Autodesk Inventor part; units mm, degrees
ref_plane "YZ Plane" through (0, 0, 0) normal (1, 0, 0) x (0, 1, 0)
ref_plane "XZ Plane" through (0, 0, 0) normal (0, 1, 0) x (-1, 0, 0)
ref_plane "XY Plane" through (0, 0, 0) normal (0, 0, 1) x (1, 0, 0)
sketch "Sketch1" plane through (0, 0, 0) normal (0, 1, 0) x (-1, 0, 0)
  line L0 (0, 0) -> (49, 0) construction
  line L1 (49, 0) -> (49, -58) construction
  line L2 (49, -58) -> (0, -58) construction
  line L3 (0, -58) -> (0, 0) construction
  line L4 (53.5, 32) -> (-4.5, 32) construction
  line L5 (-4.5, 32) -> (-4.5, -62) construction
  line L6 (-4.5, -62) -> (53.5, -62) construction
  line L7 (53.5, -62) -> (53.5, 32) construction
  line L8 (53.5, -58) -> (-4.5, -58) construction
  line L9 (24.5, -62) -> (24.5, -133) construction
  line L10 (49, -70.5) -> (28, -70.5) construction
  line L11 (28, -70.5) -> (28, -127.5) construction
  line L12 (28, -127.5) -> (49, -127.5) construction
  line L13 (49, -127.5) -> (49, -70.5) construction
  line L14 (24.5, -99) -> (28, -99) construction
  line L15 (45.5, -127.5) -> (31.5, -127.5) construction
  line L16 (31.5, -127.5) -> (31.5, -140.5) construction
  line L17 (31.5, -140.5) -> (45.5, -140.5) construction
  line L18 (45.5, -140.5) -> (45.5, -127.5) construction
  line L19 (16.5, -82.13) -> (0, -82.13) construction
  line L20 (0, -82.13) -> (0, -112.87) construction
  line L21 (0, -112.87) -> (16.5, -112.87) construction
  line L22 (16.5, -112.87) -> (16.5, -82.13) construction
  line L23 (24.5, -97.5) -> (16.5, -97.5) construction
  circle A0 centre (49, -127.5) radius 1.5
  circle A1 centre (49, -70.5) radius 1.5
  circle A2 centre (28, -70.5) radius 1.5
  circle A3 centre (28, -127.5) radius 1.5
  circle A4 centre (49, -58) radius 1.5
  circle A5 centre (0, -58) radius 1.5
  circle A6 centre (0, 0) radius 1.5
  circle A7 centre (49, 0) radius 1.5
  circle A8 centre (16.5, -82.13) radius 1.5
  circle A9 centre (0, -112.87) radius 1.5
  line L24 (53.5, 32) -> (-4.5, 32) construction
  line L25 (-4.5, 32) -> (-4.5, -140.5) construction
  line L26 (-4.5, -140.5) -> (53.5, -140.5) construction
  line L27 (53.5, -140.5) -> (53.5, 32) construction
  line L28 (56.5, 35) -> (-7.5, 35) construction
  line L29 (-7.5, 35) -> (-7.5, -143.5)
  line L30 (-7.5, -143.5) -> (56.5, -143.5) construction
  line L31 (56.5, -143.5) -> (56.5, 35)
  arc A10 (56.5, 35) -> (-7.5, 35) centre (24.5, 35) ccw
  arc A11 (-7.5, -143.5) -> (56.5, -143.5) centre (24.5, -143.5) ccw
  point P0 (24.5, -58)
  point P1 (38.5, -127.5)
  point P2 (38.5, -140.5)
  point P3 (53.5, -15)
  point P4 (-4.5, -15)
  point P5 (24.5, 32)
  dimension "d0" = 49
  dimension "d1" = 58
  dimension "d2" = 58
  dimension "d3" = 94
  dimension "d7" = 71
  dimension "d8" = 21
  dimension "d9" = 57
  dimension "d10" = 37
  dimension "d11" = 3.5
  dimension "d12" = 14
  dimension "d13" = 13
  dimension "d14" = 16.5
  dimension "d15" = 30.74
  dimension "d16" = 8
  dimension "d17" = 3
  dimension "d18" = 3
  dimension "d19" = 3
  dimension "d20" = 3
  dimension "d21" = 3
  dimension "d22" = 3
  dimension "d23" = 3
  dimension "d24" = 3
  dimension "d25" = 3
  dimension "d26" = 3
  dimension "d27" = 3
  dimension "d43" = 4
extrude "Extrusion1" add sketch "Sketch1" along normal blind 3
sketch "Sketch2" plane through (0, 0, 0) normal (0, -1, 0) x (1, 0, 0)
  arc A0 (-56.5, -143.5) -> (7.5, -143.5) centre (-24.5, -143.5) ccw
  line L0 (7.5, 35) -> (7.5, -143.5)
  arc A1 (7.5, 35) -> (-56.5, 35) centre (-24.5, 35) ccw
  line L1 (-56.5, -143.5) -> (-56.5, 35)
  circle A2 centre (0, -112.87) radius 1.5
  circle A3 centre (-49, 0) radius 1.5
  circle A4 centre (0, 0) radius 1.5
  circle A5 centre (0, -58) radius 1.5
  circle A6 centre (-49, -58) radius 1.5
  circle A7 centre (-28, -127.5) radius 1.5
  circle A8 centre (-28, -70.5) radius 1.5
  circle A9 centre (-49, -70.5) radius 1.5
  circle A10 centre (-49, -127.5) radius 1.5
  circle A11 centre (-16.5, -82.13) radius 1.5
  circle A12 centre (0, 0) radius 3.5
  circle A13 centre (-49, 0) radius 3.5
  circle A14 centre (-49, -58) radius 3.5
  circle A15 centre (0, -58) radius 3.5
  circle A16 centre (-28, -70.5) radius 3.5
  circle A17 centre (-49, -70.5) radius 3.5
  circle A18 centre (-16.5, -82.13) radius 3.5
  circle A19 centre (0, -112.87) radius 3.5
  circle A20 centre (-28, -127.5) radius 3.5
  circle A21 centre (-49, -127.5) radius 3.5
  dimension "d31" = 2
  dimension "d32" = 2
  dimension "d33" = 2
  dimension "d34" = 2
  dimension "d35" = 2
  dimension "d36" = 2
  dimension "d37" = 2
  dimension "d38" = 2
  dimension "d39" = 2
  dimension "d40" = 2
extrude "Extrusion2" cut sketch "Sketch2" against normal blind 2 contours A12 | A13 | A14 | A15 | A16 | A17 | A18 | A19 | A20 | A21
sketch "Sketch3" plane through (0, 3, 0) normal (0, 1, 0) x (1, 0, 0)
  arc A0 (-56.5, -35) -> (7.5, -35) centre (-24.5, -35) ccw
  circle A1 centre (-24.5, -67) radius 4.9
  arc A2 (7.5, 143.5) -> (-56.5, 143.5) centre (-24.5, 143.5) ccw
  circle A3 centre (-24.5, 175.5) radius 4.9
  point P0 (0, 0)
  point P1 (-29.3856, 175.1248)
  point P2 (-19.6144, 175.1248)
  point P3 (-19.6144, -66.6248)
  point P4 (-29.3856, -66.6248)
  dimension "d44" = 9.8
  dimension "d45" = 9.8
extrude "Extrusion3" cut sketch "Sketch3" against normal through all contours A1 A0 | A3 A2 picked at (-24.5, -65.3388) picked at (-24.5, 173.8388)
properties part number "electronics_layout_v2"
The listing builds one solid part. Answer for the finished solid, in the listing's coordinates (mm). A direction names the side the tool comes from. Round coordinates to 2 decimals unless told otherwise and drop trailing zeros. Order: outer loops, then holes, each group sorted by start corner. A loop starts at its lowest first (then second) coordinate and runs counter-clockwise, first axis right, second up. Notation, with made-up numbers: (80.5, 13) -> (121.5, 13) arc R17 cw to (121.5, 20) -> close; hole circle Ø1 at (-13.5, 71.5). An arc over 180 degrees is marked (long way). Answer as CSV lines item,"result". Start each with the question number.
(1) The part is cut by section B-B (x = -6). Determine the outline of the cut face in (y, z), then the cut area to 3 significant figures.
(2) For a pull along Z with two mould halves and no side action, classify faces 1 (the face through (-24.6, 1.5, -170.6)), 2 (the face through (-14.62, 0.99, -79.18)), 3 (the face through (-24, 3, -53)), 4 (the face through (-48.586, 1.479, 56.069)) as +Z half, -Z half, draft (parallel to the pull), parting line (faces both ways), or undercut.
(3) The part is cut by section A-A (y = 1.5). Count the separate pieces of the cut face and the enclosed holes in it, then the cut area to 3 significant figures.
(4) Find the intervals of material crossed by probe 1 along X at (y, z) = (2.65, 0); probe 2 along Z at (x, y) = (0, 2.7); probe 3 along Z at (x, y) = (-49, 0.7), in increasing order. Write a range as from..to.
(5) Flat-ended cylindrical pins translate along their axes: pin 1 Ø6.5 at (x, z) = (-16.5, -82.13) entering from -Y; pin 2 Ø1 at (y, z) = (2.5, 36.5) entering from -X; pin 3 Ø1.5 at (x, y) = (-47.5, 1) entering from +Z. Find the tip coordinate at first contact, or state that the pin passes through.
(6) A tool of negligible diameter and unlimited length cuts with its end or side. For faces 5 (the face through (-17, 2, -84)), 6 (the face through (-0.414, 1.479, -164.569)), from which of +Z, -Z, +X, -X, +Y, -Y can it reach the whole face along a straight path? Write none if from no direction.
Evaluation:
1,outline,"(0, -169.61) -> (3, -169.61) -> (3, 61.11) -> (0, 61.11) -> close"
1,area,"692 mm²"
2,face 1,"-Z half"
2,face 2,"undercut"
2,face 3,"draft"
2,face 4,"+Z half"
3,separate pieces,"1"
3,enclosed holes,"10"
3,area,"14,200 mm²"
4,probe 1,"-56.5..-50.5, -47.5..-1.5, 1.5..7.5"
4,probe 2,"-164.09..-114.37, -111.37..-59.5, -56.5..-1.5, 1.5..55.59"
4,probe 3,"-164.09..-131, -124..-74, -67..-61.5, -54.5..-3.5, 3.5..55.59"
5,pin 1,"y = 2"
5,pin 2,"x = -56.48"
5,pin 3,"z = 58"
6,face 5,"-Y"
6,face 6,"-Z, +X, +Y, -Y"
